Geometry check sheet. Reference: the model listing, model coordinates, mm. A direction names the side the tool comes from. Round coordinates to 2 decimals unless told otherwise and drop trailing zeros. Write each loop counter-clockwise with the first axis right and the second up, starting at its lowest first coordinate (ties: lowest second). Pieces come first, ordered by that corner, then holes.
Item 1: Cross-section at C-C (z = 6.25). Enter the section's corners in (x, y), then the cut area to 3 significant figures.
Item 2: Cross-section at D-D (y = -6.75). Enter the section's corners in (x, z).
Item 3: Scan lines: probe 1 along X at (y, z) = (-3.5, 11.5); probe 2 along Y at (x, z) = (3.5, 10.5); probe 3 along Z at (x, y) = (0, -8.25). Record each from-to range of solid material in increasing order.
Item 4: Cross-section at A-A (y = -0.5). Enter the section's corners in (x, z), then the cut area to 4 significant figures.
Item 5: Depth check by flat-ended pin: P1, Ø4, axis at y = 3.5, z = 8, coming from the -X side; P2, Ø1, axis at y = -3.5, z = 2.5, coming from the +X side; P3, Ø1, axis at x = 5, y = -3.5, coming from the -Z side; P4, Ø1.6, axis at x = -6.5, z = -0.5, coming from the -Y side. Enter the tip coordinate at first touch or a pass-through.
Item 6: Access from +Z, -Z, +X, -X, +Y, -Y to the whole of each face (thin tool, end or side, straight path). Record for faces 1 (the face through (4.706, -5.076, 8.318)), 2 (the face through (3, -6.21, 8)), 3 (the face through (1.32, 1, 8)), 4 (the face through (-3.5, 0, -1)).
Item 7: Cross-section at B-B (x = -6.25). Enter the section's corners in (y, z), then the cut area to 3 significant figures.
from build123d import *

# Parameters (mm, degrees)
SKETCH_W     = 16
SKETCH_H     = 18.5
PAD_DEPTH    = 1.6
FILLET_R     = 1
SKETCH001_W  = 4.4
SKETCH001_H  = 13.7
PAD001_DEPTH = 13.25
POCKET_DEPTH = 13.25
SKETCH003_W  = 4.5
SKETCH003_H  = 14.66
PAD002_DEPTH = 1.5


with BuildPart() as part:
    # Sketch → Pad (new body)
    with BuildSketch(Plane.XY):
        Rectangle(SKETCH_W, SKETCH_H)
    extrude(amount=PAD_DEPTH)

    # Fillet
    fillet_edges = [part.edges().sort_by_distance(p)[0] for p in [
        (8, -9.25, 0.8),
        (-8, -9.25, 0.8),
        (-8, 9.25, 0.8),
        (8, 9.25, 0.8),
    ]]
    fillet(fillet_edges, radius=FILLET_R)

    # Sketch001 (on Face5 of Fillet) → Pad001 (join)
    with BuildSketch(Plane.XY.offset(1.6)):
        with Locations((3.52, 0.64)):
            Rectangle(SKETCH001_W, SKETCH001_H)
    extrude(amount=PAD001_DEPTH)

    # Sketch002 (on Face15 of Pad001) → Pocket (cut)
    with BuildSketch(Plane.XY.offset(14.85)):
        Polygon((5.72, 7.49), (5.72, 5.19), (3.72, 7.49), align=None)
        Polygon((5.72, -3.91), (5.72, -6.21), (3.72, -6.21), align=None)
    extrude(amount=-POCKET_DEPTH, mode=Mode.SUBTRACT)

    # Sketch003 (on Face2 of Pocket) → Pad002 (join)
    with BuildSketch(Plane(origin=(0, 0, 0), x_dir=(1, 0, 0), z_dir=(0, 0, -1))):
        with Locations((-5.75, 0)):
            Rectangle(SKETCH003_W, SKETCH003_H)
    extrude(amount=PAD002_DEPTH)


solid = part.part
Resolved:
1. outline: (1.32, -6.21) - (3.72, -6.21) - (5.72, -3.91) - (5.72, 5.19) - (3.72, 7.49) - (1.32, 7.49) - close
1. area: 55.7 mm2
2. outline: (-8, -1.5) - (-3.5, -1.5) - (-3.5, 0) - (8, 0) - (8, 1.6) - (-8, 1.6) - close
3. probe 1: x = 1.32 to 5.72
3. probe 2: y = -6.21 to 7.49
3. probe 3: z = 0 to 1.6
4. outline: (-8, -1.5) - (-3.5, -1.5) - (-3.5, 0) - (8, 0) - (8, 1.6) - (5.72, 1.6) - (5.72, 14.85) - (1.32, 14.85) - (1.32, 1.6) - (-8, 1.6) - close
4. area: 90.65 mm2
5. P1: stops at x = 1.32
5. P2: stops at x = 5.72
5. P3: stops at z = 0
5. P4: stops at y = -9.25
6. face 1: +Z, +X, -Y
6. face 2: +Z, +X, -X, -Y
6. face 3: +Z, -X, +Y, -Y
6. face 4: -Z, +X, +Y, -Y
7. outline: (-9.25, 0) - (-7.33, 0) - (-7.33, -1.5) - (7.33, -1.5) - (7.33, 0) - (9.25, 0) - (9.25, 1.6) - (-9.25, 1.6) - close
7. area: 51.6 mm2
